For this review, take the finished solid that the model builds, in its own axes (mm). A direction names the side the tool comes from. Round coordinates to 2 decimals unless told otherwise and drop trailing zeros. Order: outer loops, then holes, each group sorted by start corner. A loop starts at its lowest first (then second) coordinate and runs counter-clockwise, first axis right, second up.
```python
from build123d import *

# Parameters (mm, degrees)
OTW_R_GWINTOWANY_M161_D = 14


# Read off the part's stored shape, not the designer's step: Obrót1
with BuildPart() as part:
    # Obrót1 outline → Obrót1 (revolve)
    with BuildSketch(Plane.XY):
        Polygon((0, 10.090604818), (0, 0), (20.5, 0), (21.5, 1), (21.5, 4.5), (21, 4.5), (21, 119), (20, 120), (17.5, 120), (16.5, 119), (16.5, 13), align=None)
    revolve(axis=Axis((0, 0, 0), (0, 1, 0)))

    # Otwór gwintowany M161 (through all)
    with Locations(Plane(origin=(0, 0, 0), x_dir=(0, 0, -1), z_dir=(0, -1, 0))):
        with Locations((0, 0)):
            Hole(OTW_R_GWINTOWANY_M161_D / 2)


solid = part.part
```
Q1. Take a section at B-B, the plane z = 0. State the section outline as (x, y) points.
Q2. Mouldability with a two-part tool opening along Z and no side actions: class faces 1 (the face through (0, 120, 18)), 2 (the face through (-2.681, 5.742, 6.466)), 3 (the face through (-2.799, 2.774, -21.317)) as +Z half, -Z half, draft (parallel to the pull), parting line (faces both ways), or undercut.
Q3. Take a section at A-A, the plane x = 0. State the section outline as (y, z) points.
Q4. Wall thickness on line 1 (X direction, y = 53, z = 0); line 2 (Z direction, x = 0, y = 7.25); line 3 (Z direction, x = 0, y = 2.5): over which ranges is each line inside the solid? List them lowest first.
Q5. Clearance check with flat-ended pins moving along their axes: pin 1 (12 mm diameter, centred on y = 55.5, z = -15, fed in from +X); pin 2 (10 mm diameter, centred on x = 6, z = -4.5, fed in from +Y); pin 3 (1.5 mm diameter, centred on y = 13, z = -13, fed in from -X). State where each tip first meets the part, or that it passes through.
Q6. Tool access review of faces 4 (the face through (19, 4.5, 9.5)), 5 (the face through (-9, 0, 0)): name each direction out of +Z, -Z, +X, -X, +Y, -Y from which nothing blocks a thin tool from reaching the whole face with its end or side.
Q7. Take a section at C-C, the plane y = 88. State the section outline as (x, z) points, plus the area to 3 significant figures.
Working result:
1. outline: (-21.5, 1) - (-20.5, 0) - (-7, 0) - (-7, 11.32) - (-16.5, 13) - (-16.5, 119) - (-17.5, 120) - (-20, 120) - (-21, 119) - (-21, 4.5) - (-21.5, 4.5) - close; (7, 0) - (20.5, 0) - (21.5, 1) - (21.5, 4.5) - (21, 4.5) - (21, 119) - (20, 120) - (17.5, 120) - (16.5, 119) - (16.5, 13) - (7, 11.32) - close
2. face 1: draft
2. face 2: undercut
2. face 3: parting line
3. outline: (0, -20.5) - (1, -21.5) - (4.5, -21.5) - (4.5, -21) - (119, -21) - (120, -20) - (120, -17.5) - (119, -16.5) - (13, -16.5) - (11.32, -7) - (0, -7) - close; (0, 7) - (11.32, 7) - (13, 16.5) - (119, 16.5) - (120, 17.5) - (120, 20) - (119, 21) - (4.5, 21) - (4.5, 21.5) - (1, 21.5) - (0, 20.5) - close
4. line 1: x = -21 to -16.5, 16.5 to 21
4. line 2: z = -21 to -7, 7 to 21
4. line 3: z = -21.5 to -7, 7 to 21.5
5. pin 1: stops at x = 18.97
5. pin 2: stops at y = 12.29
5. pin 3: stops at x = -17.06
6. face 4: +Y
6. face 5: +Z, -Z, +X, -X, -Y
7. outline: circle Ø42 at (0, 0); hole circle Ø33 at (0, 0)
7. area: 530 mm2
